Input: part model. Units: mm. Frame: model coordinates. A direction names the side the tool comes from. Coordinates: 2 decimals unless noted, no trailing zeros. Write each loop counter-clockwise with the first axis right and the second up, starting at its lowest first coordinate (ties: lowest second). Pieces come first, ordered by that corner, then holes.
1) Section query B-B (x = 28). Output: boundary loops of the cut face in (y, z) (3 decimals), then the cut area to 3 significant figures.
2) Section query D-D (x = 2). Output: boundary loops of the cut face in (y, z) (3 decimals).
3) Set-up query: faces 1 (the flat face through (-29.339, -0.044, -34.816)), 2 (the flat face through (33.858, 0, -25)), 3 (the cylindrical face through (13.92, -0.04, -26.35)). Return all of +Z, -Z, +X, -X, +Y, -Y with unobstructed straight access to the full face (end or side cutting, diameter ignored); none if empty.
4) Line query: L1, parallel to X at y = 2.5, z = -22; L2, parallel to X at y = -1, z = -2.5; L3, parallel to X at y = 0, z = -14. Output: solid intervals per line, ascending.
5) Pin query (flat end, axial travel): pin 1 Ø1.7 at (x, z) = (-17.3, -2.551) entering from +Y; pin 2 Ø4 at (x, z) = (17.3, 19.449) entering from +Y (3 decimals). Return the tip coordinate at first contact, or that it passes through.
6) Section query A-A (z = -13.5). Output: boundary loops of the cut face in (x, y) (3 decimals), then the cut area to 3 significant figures.
7) Section query C-C (y = 1). State how many separate pieces and enclosed holes the cut face has, then the cut area to 3 significant figures.
8) Draft query along X for faces 4 (the cylindrical face through (30.554, 0.044, -30.365)), 5 (the flat face through (-38.1, 0, -2)), 6 (the flat face through (-17, 3.175, -6)). Return one class per face: pulls with the +X half, pulls with the -X half, needs draft (parallel to the pull), parting line crosses it, or undercut.
from build123d import *

# Parameters (mm, degrees)
SKETCH1_W              = 76.2
SKETCH1_H              = 76.2
BOSS_EXTRUDE1_DEPTH    = 3.175
SKETCH2_W              = 29.6545
SKETCH2_H              = 54.61
CUT_EXTRUDE1_DEPTH     = 55.254423783
M2_5_CLEARANCE_HOLE1_D = 2.9
CUT_EXTRUDE2_DEPTH     = 55.254423783
SKETCH9_W              = 76.2
SKETCH9_H              = 10.795
SKETCH9_H_2            = 0.41
CUT_EXTRUDE3_DEPTH     = 55.254423783
CUT_EXTRUDE4_DEPTH     = 54.967291946
FILLET1_R              = 3.175


with BuildPart() as part:
    # Sketch1 → Boss-Extrude1 (new, symmetric)
    with BuildSketch(Plane(origin=(0, 0, 0), x_dir=(1, 0, 0), z_dir=(0, 1, 0))):
        Rectangle(SKETCH1_W, SKETCH1_H)
    extrude(amount=BOSS_EXTRUDE1_DEPTH, both=True)

    # Sketch2 → Cut-Extrude1 (cut, through all)
    with BuildSketch(Plane(origin=(0, 3.175, 0), x_dir=(1, 0, 0), z_dir=(0, 1, 0))):
        Rectangle(SKETCH2_W, SKETCH2_H)
    extrude(amount=-CUT_EXTRUDE1_DEPTH, mode=Mode.SUBTRACT)

    # M2.5 Clearance Hole1 (through all)
    with Locations(Plane(origin=(0, 3.175, 0), x_dir=(1, 0, 0), z_dir=(0, 1, 0))):
        with Locations((-17.3, 24.551), (-11, 29.851), (-17.3, 2.551), (-17.3, -19.449)):
            m2_5_clearance_hole1 = Hole(M2_5_CLEARANCE_HOLE1_D / 2)

    # Sketch8 → Cut-Extrude2 (cut, through all)
    with BuildSketch(Plane(origin=(0, 3.175, 0), x_dir=(1, 0, 0), z_dir=(0, 1, 0))):
        with BuildLine():
            Line((-33.8582, -14.2875), (-33.8582, -11.1125))
            ThreePointArc((-33.8582, -11.1125), (-30.48, -7.7343), (-27.1018, -11.1125))
            Line((-27.1018, -11.1125), (-27.1018, -14.2875))
            ThreePointArc((-27.1018, -14.2875), (-30.48, -17.6657), (-33.8582, -14.2875))
        make_face()
        with BuildLine():
            Line((-33.8582, 23.8125), (-33.8582, 26.9875))
            ThreePointArc((-33.8582, 26.9875), (-30.48, 30.3657), (-27.1018, 26.9875))
            Line((-27.1018, 26.9875), (-27.1018, 23.8125))
            ThreePointArc((-27.1018, 23.8125), (-30.48, 20.4343), (-33.8582, 23.8125))
        make_face()
    cut_extrude2 = extrude(amount=-CUT_EXTRUDE2_DEPTH, mode=Mode.SUBTRACT)

    # Mirror1: M2.5 Clearance Hole1, Cut-Extrude2 across plane
    add(m2_5_clearance_hole1.mirror(Plane(origin=(0, 0, 0), x_dir=(0, 0, 1), z_dir=(1, 0, 0))), mode=Mode.SUBTRACT)
    add(cut_extrude2.mirror(Plane(origin=(0, 0, 0), x_dir=(0, 0, 1), z_dir=(1, 0, 0))), mode=Mode.SUBTRACT)

    # Sketch9 → Cut-Extrude3 (cut, through all)
    with BuildSketch(Plane(origin=(0, 3.175, 0), x_dir=(1, 0, 0), z_dir=(0, 1, 0))):
        with Locations((0, -32.7025)):
            Rectangle(SKETCH9_W, SKETCH9_H)
        with Locations((0, 37.895)):
            Rectangle(SKETCH9_W, SKETCH9_H_2)
    extrude(amount=-CUT_EXTRUDE3_DEPTH, mode=Mode.SUBTRACT)

    # Sketch13 → Cut-Extrude4 (cut, through all)
    with BuildSketch(Plane.XZ.offset(3.175)):
        Polygon((-38.1, -31.213), (-22.352, -37.69), (-38.1, -37.69), align=None)
    cut_extrude4 = extrude(amount=-CUT_EXTRUDE4_DEPTH, mode=Mode.SUBTRACT)

    # Mirror3: Cut-Extrude4 across plane
    add(cut_extrude4.mirror(Plane(origin=(0, 0, 0), x_dir=(0, 0, 1), z_dir=(1, 0, 0))), mode=Mode.SUBTRACT)

    # Fillet1
    fillet1_edges = [part.edges().sort_by_distance(p)[0] for p in [
        (-38.1, 0, 27.305),
        (38.1, 0, 27.305),
        (-38.1, 0, -31.213),
        (14.82725, 0, -27.305),
        (38.1, 0, -31.213),
        (14.82725, 0, 27.305),
        (-14.82725, 0, 27.305),
        (-14.82725, 0, -27.305),
    ]]
    fillet(fillet1_edges, radius=FILLET1_R)


solid = part.part
Answer:
1. outline: (-3.175, -35.367) - (3.175, -35.367) - (3.175, -29.281) - (-3.175, -29.281) - close; (-3.175, -21.519) - (3.175, -21.519) - (3.175, 8.819) - (-3.175, 8.819) - close; (-3.175, 16.581) - (3.175, 16.581) - (3.175, 27.305) - (-3.175, 27.305) - close
1. area: 299 mm2
2. outline: (-3.175, -37.69) - (3.175, -37.69) - (3.175, -27.305) - (-3.175, -27.305) - close
3. face 1: -Z, -X, +Y, -Y
3. face 2: +Y, -Y
3. face 3: +Z, +Y, -Y
4. L1: x = -38.1 to -33.33, -27.63 to -14.83, 14.83 to 27.63, 33.33 to 38.1
4. L2: x = -38.1 to -18.75, -15.85 to -14.83, 14.83 to 15.85, 18.75 to 38.1
4. L3: x = -38.1 to -14.83, 14.83 to 38.1
5. pin 1: passes through
5. pin 2: stops at y = 3.175
6. outline: (-38.1, -3.175) - (-14.827, -3.175) - (-14.827, 3.175) - (-38.1, 3.175) - close; (14.827, -3.175) - (38.1, -3.175) - (38.1, 3.175) - (14.827, 3.175) - close
6. area: 296 mm2
7. separate pieces: 1
7. enclosed holes: 12
7. area: 2,940 mm2
8. face 4: undercut
8. face 5: pulls with the -X half
8. face 6: needs draft
